Verification items for this drawing (mm, ordinates from the low corner). Give positions to 0.01 mm unless a question says otherwise; leave off trailing zeros. Order: outer loops, then holes, each group sorted by start corner. A loop starts at its lowest first (then second) coordinate and runs counter-clockwise, first axis right, second up. Notation, with made-up numbers: (58, -37) -> (92, -37) arc R24 ccw to (92, -5) -> close; hole circle Ø2 at (15, 68). An arc over 180 degrees is marked (long way). One line per question, with ' | ' between items.
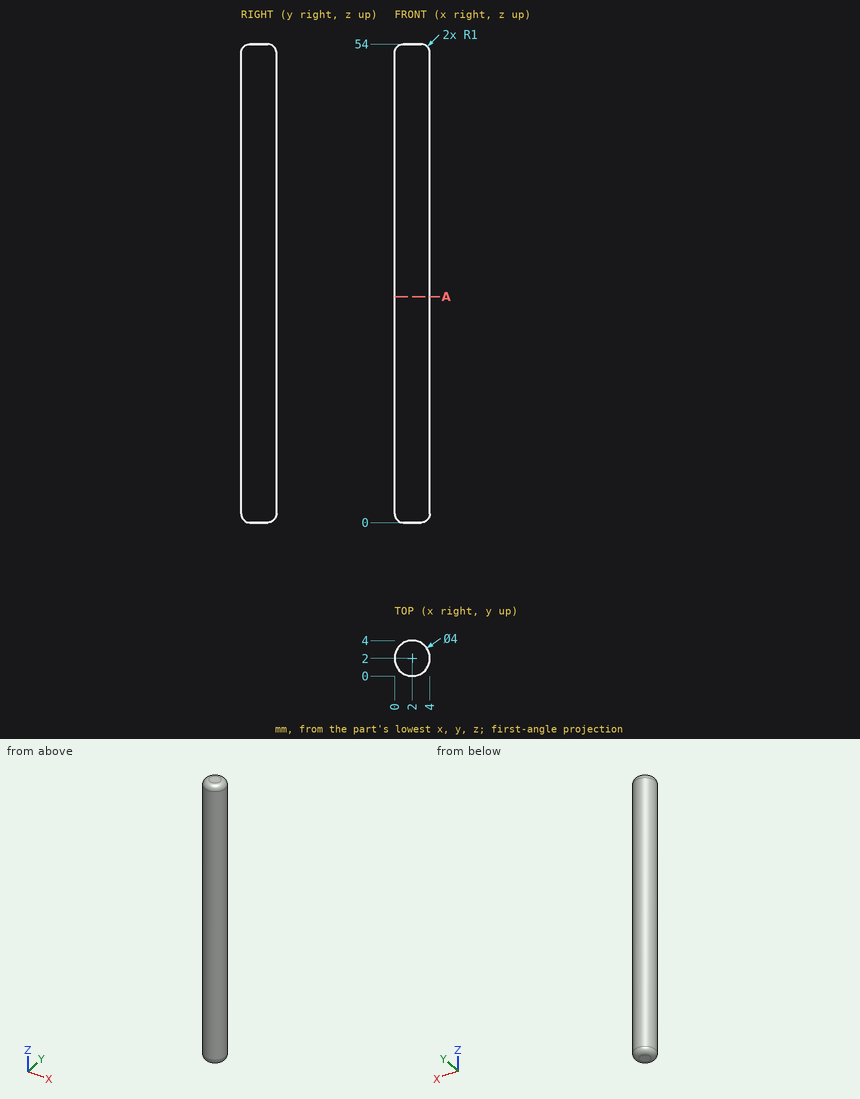
Q1. Depth check by flat-ended pin: pin 1 Ø1.5 at (y, z) = (1, 28) entering from -X. Enter the tip coordinate at first touch or a pass-through.
Result sheet:
pin 1: stops at x = 0.02
Q2. Thickness scan on line 1 (Y direction, x = 1.85, z = 17); line 2 (Y direction, x = 2.5, z = 30.5); line 3 (X direction, y = 3.3, z = 8). Record the ranges inside material, lowest first.
Result sheet:
line 1: y = 0.01 to 3.99 | line 2: y = 0.06 to 3.94 | line 3: x = 0.48 to 3.52
Q3. Section check A-A (z = 25.5). Enter the section's corners in (x, y).
Result sheet:
outline: circle Ø4 at (2, 2)
